Verification items for the finished model (mm, model axes). Face numbers are marked on the shaded views. A direction names the side the tool comes from. Coordinates: 2 decimals unless noted, no trailing zeros. Write each loop counter-clockwise with the first axis right and the second up, starting at its lowest first coordinate (ties: lowest second). Pieces come first, ordered by that corner, then holes.
Autodesk Inventor part; units mm, degrees
ref_plane "YZ Plane" through (0, 0, 0) normal (1, 0, 0) x (0, 1, 0)
ref_plane "XZ Plane" through (0, 0, 0) normal (0, 1, 0) x (-1, 0, 0)
ref_plane "XY Plane" through (0, 0, 0) normal (0, 0, 1) x (1, 0, 0)
sketch "Sketch1" plane through (0, 0, 0) normal (1, 0, 0) x (0, 1, 0)
  line L0 (0, 0) -> (0, -38.1)
  line L1 (0, -38.1) -> (68.58, -38.1)
  line L2 (68.58, -38.1) -> (68.58, -28.956)
  line L3 (68.58, -28.956) -> (6.35, -28.956)
  line L4 (0, 0) -> (12.7, 0)
  line L5 (12.7, 0) -> (12.7, -6.35)
  line L6 (12.7, -6.35) -> (6.35, -6.35)
  line L7 (0, 0) -> (6.35, 0)
  line L8 (6.35, -6.35) -> (6.35, -28.956)
  line L9 (68.58, -38.1) -> (48.26, -38.1)
  line L10 (48.26, -38.1) -> (48.26, 0)
  line L11 (48.26, 0) -> (68.58, 0)
  line L12 (68.58, 0) -> (68.58, -38.1)
  dimension "d0" = 38.1
  dimension "d1" = 68.58
  dimension "d2" = 9.144
  dimension "d3" = 6.35
  dimension "d4" = 12.7
  dimension "d5" = 6.35
  dimension "d6" = 6.35
  dimension "d10" = 20.32
  dimension "d11" = 38.1
extrude "Extrusion2" add sketch "Sketch1" along normal blind 9.398
sketch "Sketch2" plane through (9.398, 0, 0) normal (1, 0, 0) x (0, 0, -1)
  line L0 (28.956, 48.26) -> (28.956, 6.35)
  line L1 (28.956, 6.35) -> (6.35, 6.35)
  line L2 (6.35, 6.35) -> (6.35, 12.7)
  line L3 (6.35, 12.7) -> (0, 12.7)
  line L4 (0, 12.7) -> (0, 0)
  line L5 (0, 0) -> (38.1, 0)
  line L6 (38.1, 0) -> (38.1, 68.58)
  line L7 (38.1, 68.58) -> (0, 68.58)
  line L8 (0, 68.58) -> (0, 48.26)
  line L9 (0, 48.26) -> (28.956, 48.26)
  point P0 (28.2575, 58.42)
  point P1 (9.8425, 58.42)
  dimension "d14" = 18.415
  dimension "d15" = 38.1
  dimension "d16" = 9.8425
  dimension "d17" = 20.32
  dimension "d18" = 10.16
  dimension "d19" = 10.16
hole "Hole1" at (9.398, 58.42, -28.2575) at (9.398, 58.42, -9.8425) direction (-1, 0, 0) diameter 3.556 depth 10.9728 tip angle 118
fillet "Fillet2" radius 6.35 3 edges at (4.699, 6.35, -6.35) (4.699, 6.35, -28.956) (4.699, 48.26, -28.956)
properties part number "hook"
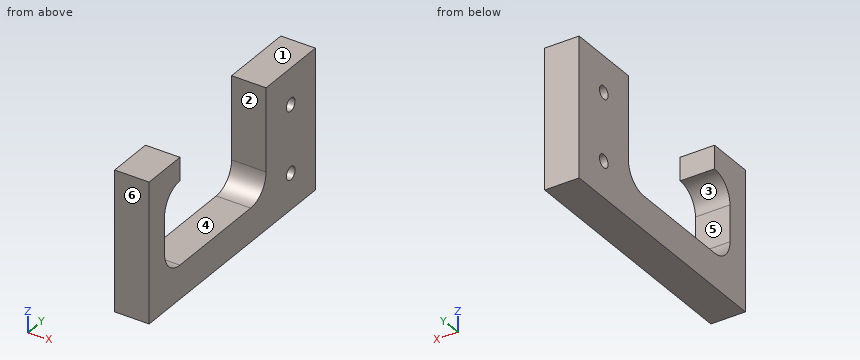
1. Sectioned sample at C-C, the plane x = 5.5. Give the number of separate pieces and of enclosed holes in the cut face, and give its area (3 significant figures).
2. Tool access check on the marked faces 1, 2 and 3. Record the directions out of +Z, -Z, +X, -X, +Y, -Y that give a thin tool (end or side, any length) a straight path to the whole face; none if there is none.
3. Draft check along Z on the marked faces 4, 5 and 6. Enter one of: pulls with the +Z half, pulls with the -Z half, needs draft (parallel to the pull), parting line crosses it, or undercut.
4. Material ranges on L1, parallel to Z at x = 3.5, y = 58.42; L2, parallel to Y at x = 5.75, z = -6; L3, parallel to Y at x = 3, z = -15, recorded low to high.
5. Sectioned sample at B-B, the plane z = -19. Record the boundary of the cut face in (x, y), and give its area (3 significant figures).
6. Sectioned sample at A-A, the plane y = 58.42. Record the boundary of the cut face in (x, z), and give its area (3 significant figures).
7. Sectioned sample at D-D, the plane z = -9. Record the boundary of the cut face in (x, y).
Outcome:
1. separate pieces: 1
1. enclosed holes: 2
1. area: 1,450 mm2
2. face 1: +Z, +X, -X, +Y, -Y
2. face 2: +Z, +X, -X
2. face 3: +X, -X
3. face 4: pulls with the +Z half
3. face 5: undercut
3. face 6: needs draft
4. L1: z = -38.1 to -30.04, -26.48 to -11.62, -8.06 to 0
4. L2: y = 0 to 12.7, 48.26 to 68.58
4. L3: y = 0 to 6.35, 48.26 to 68.58
5. outline: (0, 0) - (9.4, 0) - (9.4, 6.35) - (0, 6.35) - close; (0, 48.26) - (9.4, 48.26) - (9.4, 68.58) - (0, 68.58) - close
5. area: 251 mm2
6. outline: (0, -38.1) - (9.4, -38.1) - (9.4, -30.04) - (0, -30.04) - close; (0, -26.48) - (9.4, -26.48) - (9.4, -11.62) - (0, -11.62) - close; (0, -8.06) - (9.4, -8.06) - (9.4, 0) - (0, 0) - close
6. area: 291 mm2
7. outline: (0, 0) - (9.4, 0) - (9.4, 7.54) - (0, 7.54) - close; (0, 48.26) - (9.4, 48.26) - (9.4, 56.85) - (0, 56.85) - close; (0, 59.99) - (9.4, 59.99) - (9.4, 68.58) - (0, 68.58) - close
